Geometry check sheet. Reference: the model listing, model coordinates, mm. Round coordinates to 2 decimals unless told otherwise and drop trailing zeros. Loops run counter-clockwise (first coordinate to the right, second up) from the corner with the lowest first, then second, coordinate; pieces in that order, holes last. Notation, with made-up numbers: (64.5, 75) -> (91.5, 75) arc R20 cw to (91.5, 114) -> close; hole circle Ø4 at (89.5, 20). An arc over 180 degrees is marked (long way). Use one line per item in the form item = value.
from build123d import *

# Parameters (mm, degrees)
F2_DEPTH = 50.8


# Not quite as in the source:
# - a variable given as a bare number and used for a length is read in inches; the dataset says mm whatever the document's units were


with BuildPart() as f2:
    # F1 (on Top) → F2 (new body)
    with BuildSketch(Plane.XY):
        Polygon((0, 98.61804), (-98.61804, 98.61804), (-98.61804, -98.61804), (92.65412, -98.61804), (92.65412, 98.61804), align=None)
        with BuildLine():
            ThreePointArc((47.81804, 0), (-46.2944321696, -11.9745772173), (41.82070094, 23.1860717313))
            ThreePointArc((41.82070094, 23.1860717313), (46.2944321696, 11.9745772173), (47.81804, 0))
        make_face(mode=Mode.SUBTRACT)
    extrude(amount=F2_DEPTH)


solid = f2.part
1. Section check A-A (x = 0). Record the boundary of the cut face in (y, z), then the cut area to 3 significant figures.
Return value:
outline = (-98.62, 0) -> (-47.82, 0) -> (-47.82, 50.8) -> (-98.62, 50.8) -> close; (47.82, 0) -> (98.62, 0) -> (98.62, 50.8) -> (47.82, 50.8) -> close
area = 5,160 mm2
2. Section check B-B (z = 36.5). Record the boundary of the cut face in (x, y).
Return value:
outline = (-98.62, -98.62) -> (92.65, -98.62) -> (92.65, 98.62) -> (-98.62, 98.62) -> close; hole circle Ø95.64 at (0, 0)
3. Material ranges on line 1 along Y through (x, z) = (0, 32); line 2 along X through (y, z) = (0, 25); line 3 along X through (y, z) = (-24.5, 28), recorded low to high.
Return value:
line_1 = -98.62 to -47.82, 47.82 to 98.62
line_2 = -98.62 to -47.82, 47.82 to 92.65
line_3 = -98.62 to -41.06, 41.06 to 92.65
4. Section check C-C (x = -27.5). Record the boundary of the cut face in (y, z), then the cut area to 3 significant figures.
Return value:
outline = (-98.62, 0) -> (-39.12, 0) -> (-39.12, 50.8) -> (-98.62, 50.8) -> close; (39.12, 0) -> (98.62, 0) -> (98.62, 50.8) -> (39.12, 50.8) -> close
area = 6,050 mm2
